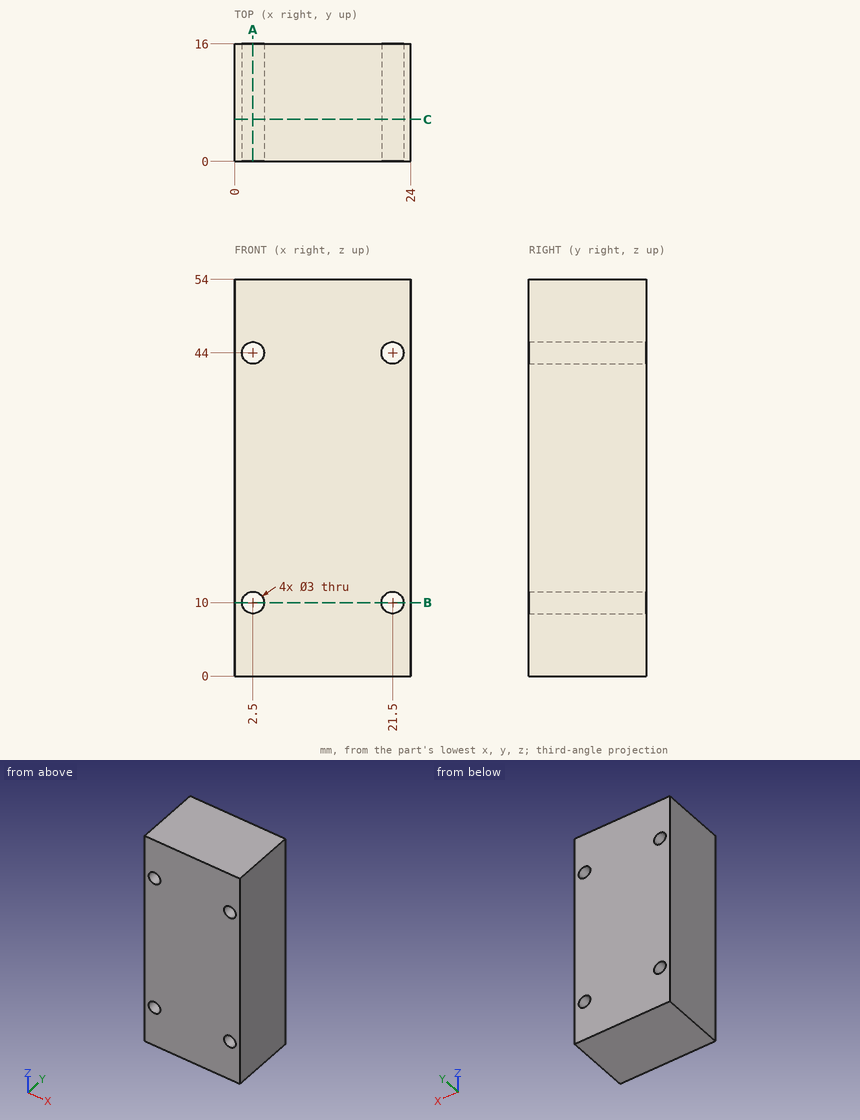
Job drawing, mm, ordinate dimensions from the low corner. One solid piece. Coordinates: 2 decimals unless noted, no trailing zeros. Order: outer loops, then holes, each group sorted by start corner. A loop starts at its lowest first (then second) coordinate and runs counter-clockwise, first axis right, second up. Notation, with made-up numbers: (49, 58.25) -> (89, 58.25) arc R25 cw to (89, 77.25) -> close; hole circle Ø10 at (51.25, 87). An arc over 180 degrees is marked (long way). Put each result on its own line as item: value. Start each with the question number.
(1) Band-saw the part on B-B (z = 10). Give the cut face in (x, y), then the cut area to 3 significant figures.
(2) Band-saw the part on A-A (x = 2.5). Give the cut face in (y, z).
(3) Band-saw the part on C-C (y = 5.75). Give the cut face in (x, z).
(4) Probe line 1 along Z through (x, y) = (21.5, 4.5); line 2 along X through (y, z) = (13.5, 10.5); line 3 along X through (y, z) = (6.25, 9). List the from-to ranges inside material, lowest first. Write a range as [from, to].
Determined:
1. outline: (0, 0) -> (1, 0) -> (1, 16) -> (0, 16) -> close; (4, 0) -> (20, 0) -> (20, 16) -> (4, 16) -> close; (23, 0) -> (24, 0) -> (24, 16) -> (23, 16) -> close
1. area: 288 mm²
2. outline: (0, 0) -> (16, 0) -> (16, 8.5) -> (0, 8.5) -> close; (0, 11.5) -> (16, 11.5) -> (16, 42.5) -> (0, 42.5) -> close; (0, 45.5) -> (16, 45.5) -> (16, 54) -> (0, 54) -> close
3. outline: (0, 0) -> (24, 0) -> (24, 54) -> (0, 54) -> close; hole circle Ø3 at (2.5, 10); hole circle Ø3 at (2.5, 44); hole circle Ø3 at (21.5, 10); hole circle Ø3 at (21.5, 44)
4. line 1: z = [0, 8.5], [11.5, 42.5], [45.5, 54]
4. line 2: x = [0, 1.09], [3.91, 20.09], [22.91, 24]
4. line 3: x = [0, 1.38], [3.62, 20.38], [22.62, 24]
